The drawing under review shows one solid part. Ordinate dimensions are in mm from its lowest x, y, z. A direction names the side the tool comes from. Coordinates: 2 decimals unless noted, no trailing zeros. Loops run counter-clockwise (first coordinate to the right, second up) from the corner with the lowest first, then second, coordinate; pieces in that order, holes last. Notation, with made-up numbers: M -6,15 L 14,15 A25 cw 14,48 Z; hole C 12.25,63 d10. An arc over 180 degrees is marked long. Answer as CSV lines item,"result". Start each with the question number.
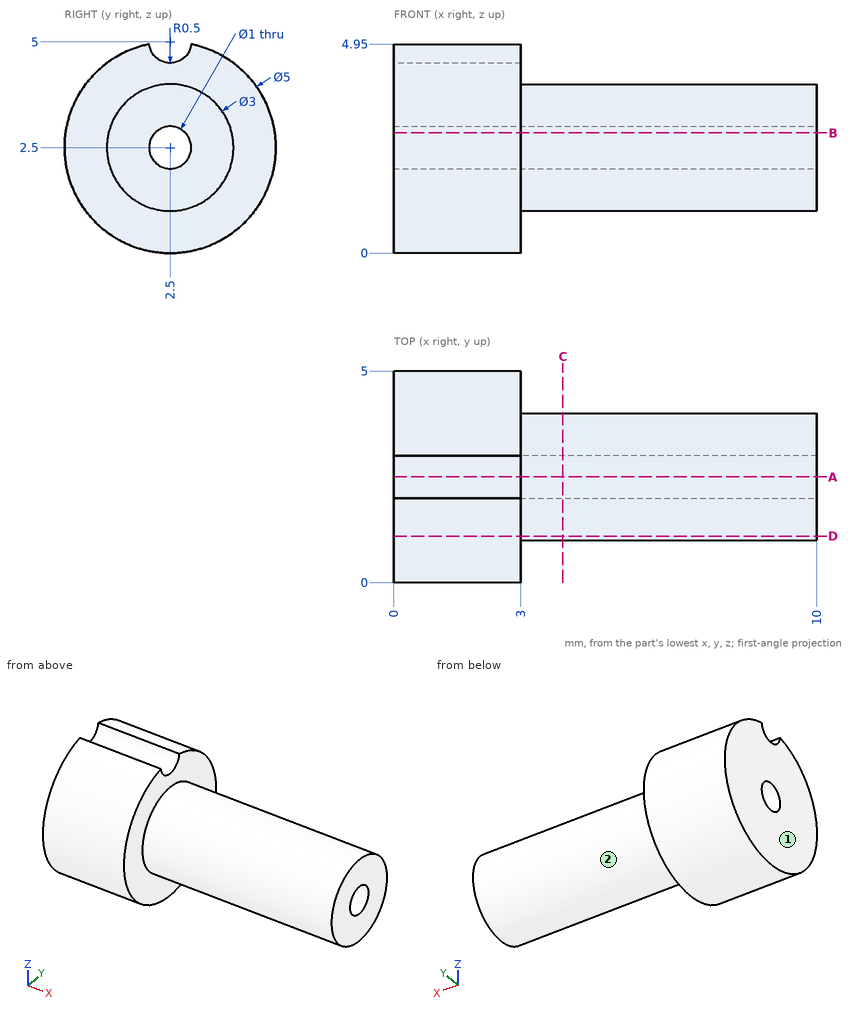
Item 1: Add section C-C (x = 4). Give the boundary of the cut face in (y, z).
Item 2: Add section A-A (y = 2.5). Give the boundary of the cut face in (x, z).
Item 3: For line 1 along Z through (x, y) = (7, 2.5); line 2 along Z through (x, y) = (2.75, 2.5); line 3 along X through (y, z) = (3.35, 4.05), list the stretches that pass through material, from the lowest coordinate up. Write a range as from..to.
Item 4: Add section D-D (y = 1.1). Give the boundary of the cut face in (x, z).
Item 5: For pin 1 (1.5 mm diameter, centred on x = 7.5, y = 2, fed in from -Z); pin 2 (2 mm diameter, centred on x = 3.5, z = 4, fed in from +Y), all flat-tipped, find the tip position at first contact; note any pin that passes through.
Item 6: Add section B-B (z = 2.85). Give the boundary of the cut face in (x, y), plus the area to 3 significant figures.
Item 7: For the marked faces 1 and 2, list the 3-axis set-ups (+Z, -Z, +X, -X, +Y, -Y) from which the entire face can be reached by the end or side of a thin tool; tool diameter is ignored.
Response:
1,outline,"C 2.5,2.5 d3; hole C 2.5,2.5 d1"
2,outline,"M 0,0 L 3,0 L 3,1 L 10,1 L 10,2 L 0,2 Z; M 0,3 L 10,3 L 10,4 L 3,4 L 3,4.5 L 0,4.5 Z"
3,line 1,"1..2, 3..4"
3,line 2,"0..2, 3..4.5"
3,line 3,"0..3"
4,outline,"M 0,0.43 L 3,0.43 L 3,1.96 L 10,1.96 L 10,3.04 L 3,3.04 L 3,4.57 L 0,4.57 Z"
5,pin 1,"z = 1"
5,pin 2,"y = 4.92"
6,outline,"M 0,0.02 L 3,0.02 L 3,1.04 L 10,1.04 L 10,2.14 L 0,2.14 Z; M 0,2.86 L 10,2.86 L 10,3.96 L 3,3.96 L 3,4.98 L 0,4.98 Z"
6,area,"28.1 mm²"
7,face 1,"+Z, -Z, -X, +Y, -Y"
7,face 2,"+X"
